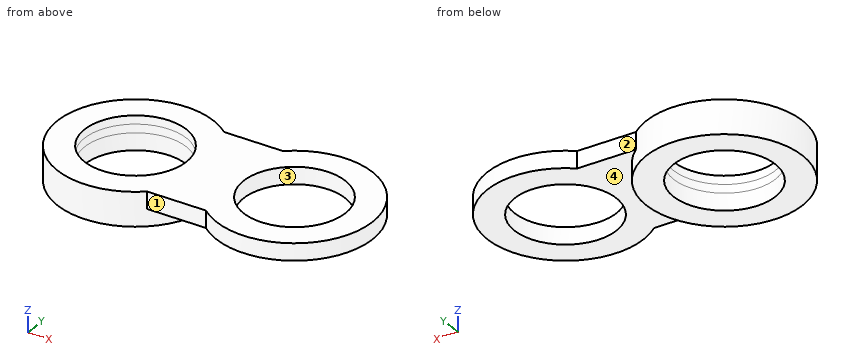
from build123d import *

# Parameters (mm, degrees)
SKETCH4_R                = 150
BOSS_EXTRUDE1_DEPTH      = 25
BOSS_EXTRUDE1_DEPTH_BACK = 25
SKETCH4_4_R              = 230
SKETCH4_4_R_2            = 150
BOSS_EXTRUDE2_DEPTH      = 75


with BuildPart() as part:
    # Sketch4 → Boss-Extrude1 (new body, two sides)
    with BuildSketch(Plane.XY) as boss_extrude1_sk:
        with BuildLine():
            Line((71.8245835, 175.909198012), (-101.8245835, 175.909198012))
            ThreePointArc((-101.8245835, 175.909198012), (-480, 0), (-101.8245835, -175.909198012))
            Line((-101.8245835, -175.909198012), (71.8245835, -175.909198012))
            ThreePointArc((71.8245835, -175.909198012), (450, 0), (71.8245835, 175.909198012))
        make_face()
        with Locations((-250, 0)):
            Circle(SKETCH4_R, mode=Mode.SUBTRACT)
        with Locations((220, 0)):
            Circle(SKETCH4_R, mode=Mode.SUBTRACT)
    extrude(amount=BOSS_EXTRUDE1_DEPTH)
    extrude(boss_extrude1_sk.sketch, amount=-BOSS_EXTRUDE1_DEPTH_BACK)

    # Sketch4_4 → Boss-Extrude2 (add)
    with BuildSketch(Plane.XY):
        with Locations((-250, 0)):
            Circle(SKETCH4_4_R)
        with Locations((-250, 0)):
            Circle(SKETCH4_4_R_2, mode=Mode.SUBTRACT)
    extrude(amount=-BOSS_EXTRUDE2_DEPTH)


solid = part.part
Can you work these out from the model? Positions are in its coordinate system, mm. Face numbers are marked on the shaded views. Give positions to 0.01 mm unless a question says otherwise; leave off trailing zeros. Order: outer loops, then holes, each group sorted by start corner. A loop starts at its lowest first (then second) coordinate and runs counter-clockwise, first axis right, second up. Notation, with made-up numbers: (-37.5, 86.5) - (12.5, 86.5) arc R14 ccw to (12.5, 93.5) - close; hole circle Ø5 at (3, -19). An arc over 180 degrees is marked (long way). Write each question's results on one line, items separated by ' | '.
1) If we mould it in two halves opening along Y, with no side actions, what happens to the marked faces 1, 2, 3 and 4? For each: pulls with the +Y half, pulls with the -Y half, needs draft (parallel to the pull), parting line crosses it, or undercut.
Final values:
face 1: pulls with the -Y half | face 2: pulls with the +Y half | face 3: undercut | face 4: needs draft
2) Suppose I cut it at C-C, the plane z = 11.5. Write out the boundary of the cut face in (x, y), then the cut area to 3 significant figures.
Final values:
outline: (-101.82, -175.91) - (71.82, -175.91) arc R230 ccw (long way) to (71.82, 175.91) - (-101.82, 175.91) arc R230 ccw (long way) to start; hole circle Ø300 at (-250, 0); hole circle Ø300 at (220, 0) | area: 212,000 mm^2
3) Suppose I cut it at D-D, the plane y = 189. Write out the boundary of the cut face in (x, z).
Final values:
outline: (-381.07, -75) - (-118.93, -75) - (-118.93, 25) - (-381.07, 25) - close; (88.93, -25) - (351.07, -25) - (351.07, 25) - (88.93, 25) - close
4) Please list where these lines run through material, in increasing order: line 1 along Y through (x, z) = (220, -11); line 2 along X through (y, z) = (20.5, -1); line 3 along Z through (x, y) = (306.5, 150.5). Write a range as [from, to].
Final values:
line 1: y = [-230, -150], [150, 230] | line 2: x = [-479.08, -398.59], [-101.41, 71.41], [368.59, 449.08] | line 3: z = [-25, 25]
5) Suppose I cut it at B-B, the plane y = 0. Write out the boundary of the cut face in (x, z), then the cut area to 3 significant figures.
Final values:
outline: (-480, -75) - (-400, -75) - (-400, 25) - (-480, 25) - close; (-100, -75) - (-20, -75) - (-20, -25) - (70, -25) - (70, 25) - (-100, 25) - close; (370, -25) - (450, -25) - (450, 25) - (370, 25) - close | area: 24,500 mm^2
6) Suppose I cut it at A-A, the plane x = -250. Write out the boundary of the cut face in (y, z).
Final values:
outline: (-230, -75) - (-150, -75) - (-150, 25) - (-230, 25) - close; (150, -75) - (230, -75) - (230, 25) - (150, 25) - close
7) I'm going to push flat-ended pins straight in: pin 1 Ø1.5 at (y, z) = (-131.5, -20.5) entering from +X; pin 2 Ø10 at (x, z) = (-280.5, -50.5) entering from +Y; pin 3 Ø5 at (y, z) = (-177.5, -64.5) entering from -X. Where does each tip first touch, or does it pass through?
Final values:
pin 1: stops at x = 409.22 | pin 2: stops at y = 228.58 | pin 3: stops at x = -399.25
